from build123d import *

# Parameters (mm, degrees)
F1_DEPTH = 32.3
F2_W     = 34
F2_H     = 43.9928
F3_DEPTH = 4.2
F4_R     = 1.8
F5_DEPTH = 25.4


with BuildPart() as f1:
    # F0 (on Top) → F1 (new body)
    with BuildSketch(Plane.XY):
        with BuildLine():
            Line((-13.075, -13.5), (13.075, -13.5))
            ThreePointArc((13.075, -13.5), (14.842766953, -12.767766953), (15.575, -11))
            Line((15.575, -11), (15.575, 11))
            ThreePointArc((15.575, 11), (14.842766953, 12.767766953), (13.075, 13.5))
            Line((13.075, 13.5), (-13.075, 13.5))
            ThreePointArc((-13.075, 13.5), (-14.842766953, 12.767766953), (-15.575, 11))
            Line((-15.575, 11), (-15.575, -11))
            ThreePointArc((-15.575, -11), (-14.842766953, -12.767766953), (-13.075, -13.5))
        make_face()
    extrude(amount=F1_DEPTH)

    # F2 (on face) → F3 (join)
    with BuildSketch(Plane.XY.offset(32.3)):
        Rectangle(F2_W, F2_H)
        with BuildLine():
            Line((-15.575, -11), (-15.575, 11))
            ThreePointArc((-15.575, 11), (-14.842766953, 12.767766953), (-13.075, 13.5))
            Line((-13.075, 13.5), (13.075, 13.5))
            ThreePointArc((13.075, 13.5), (14.842766953, 12.767766953), (15.575, 11))
            Line((15.575, 11), (15.575, -11))
            ThreePointArc((15.575, -11), (14.842766953, -12.767766953), (13.075, -13.5))
            Line((13.075, -13.5), (-13.075, -13.5))
            ThreePointArc((-13.075, -13.5), (-14.842766953, -12.767766953), (-15.575, -11))
        make_face(mode=Mode.SUBTRACT)
        with BuildLine():
            ThreePointArc((-13.075, 13.5), (-14.842766953, 12.767766953), (-15.575, 11))
            Line((-15.575, 11), (-15.575, -11))
            ThreePointArc((-15.575, -11), (-14.842766953, -12.767766953), (-13.075, -13.5))
            Line((-13.075, -13.5), (13.075, -13.5))
            ThreePointArc((13.075, -13.5), (14.842766953, -12.767766953), (15.575, -11))
            Line((15.575, -11), (15.575, 11))
            ThreePointArc((15.575, 11), (14.842766953, 12.767766953), (13.075, 13.5))
            Line((13.075, 13.5), (-13.075, 13.5))
        make_face()
    extrude(amount=F3_DEPTH)

    # F4 (on face) → F5 (cut)
    with BuildSketch(Plane.XY.offset(36.5)):
        with Locations((0, 18.0036)):
            Circle(F4_R)
        with Locations((0, -17.9964)):
            Circle(F4_R)
    extrude(amount=-F5_DEPTH, mode=Mode.SUBTRACT)


solid = f1.part
Can you work these out from the model? Positions are in its coordinate system, mm. A direction names the side the tool comes from. Coordinates: 2 decimals unless noted, no trailing zeros. Loops run counter-clockwise (first coordinate to the right, second up) from the corner with the lowest first, then second, coordinate; pieces in that order, holes last. Notation, with made-up numbers: (75, 3.5) - (114, 3.5) arc R15 cw to (114, 28.5) - close; hole circle Ø6 at (15, 88.5). An arc over 180 degrees is marked (long way). Answer as a JSON object with one key per item and string values. Group by question number.
Item 1: If I drill on L1, parallel to Y at x = 0, z = 34.6; L2, parallel to Z at x = -1.5, y = 16; L3, parallel to Y at x = 1.5, z = 28.5, over which ranges is the centre line in solid material (lowest first)? Write a range as from..to.
Item 2: On a 3-axis mill with a long thin cutter (end or side, diameter ignored), from which of +Z, -Z, +X, -X, +Y, -Y can I reach the whole of each face in a straight line? I mean faces 4 (the face through (14.82, -12.79, 15.92)), 5 (the face through (0, -13.5, 16)), 6 (the face through (0, 13.5, 16)), 7 (the face through (-15.575, 0, 16)), 8 (the face through (15.575, 0, 16)). Say none if no direction works.
Item 3: If we section it at C-C (z = 11): List the corners of the cut face in (x, y) for me (3 decimals), plus the area to 3 significant figures.
Item 4: For pin 1 (1 mm diameter, centred on x = 11.5, z = 28.5, fed in from -Y); pin 2 (8 mm diameter, centred on y = 12.5, z = 19.5, fed in from -X) (3 decimals); pin 3 (1.5 mm diameter, centred on x = -0.5, z = 24.5, fed in from +Y), each with a flat end and sliding along its axis, tell me the tip position at first contact or that it passes through.
Item 5: If we section it at A-A (x = 0): List the corners of the cut face in (y, z) for me.
Item 6: If we mould it in two halves opening along X, with no side actions, what happens to faces 1 (the face through (17, 0, 34)), 2 (the face through (0, 15, 32.3)), 3 (the face through (-0.23, -16.21, 34.43))? For each: released by +X, released by -X, zero draft, split by the parting line, or undercut.
Item 7: If we section it at B-B (x = 12.5): List the corners of the cut face in (y, z) for me, plus the area to 3 significant figures.
Returned:
{
 "1": {"L1": "y = -22..-19.8, -16.2..16.2, 19.8..22", "L2": "z = 32.3..36.5", "L3": "y = -13.5..13.5"},
 "2": {"face 4": "-Z, +X, -Y", "face 5": "-Z, +X, -X, -Y", "face 6": "-Z, +X, -X, +Y", "face 7": "-Z, -X, +Y, -Y", "face 8": "-Z, +X, +Y, -Y"},
 "3": {"outline": "(-15.575, -11) arc R2.5 ccw to (-13.075, -13.5) - (13.075, -13.5) arc R2.5 ccw to (15.575, -11) - (15.575, 11) arc R2.5 ccw to (13.075, 13.5) - (-13.075, 13.5) arc R2.5 ccw to (-15.575, 11) - close", "area": "836 mm²"},
 "4": {"pin 1": "stops at y = -13.5", "pin 2": "stops at x = -15.575", "pin 3": "stops at y = 13.5"},
 "5": {"outline": "(-22, 32.3) - (-19.8, 32.3) - (-19.8, 36.5) - (-22, 36.5) - close; (-16.2, 32.3) - (-13.5, 32.3) - (-13.5, 0) - (13.5, 0) - (13.5, 32.3) - (16.2, 32.3) - (16.2, 36.5) - (-16.2, 36.5) - close; (19.8, 32.3) - (22, 32.3) - (22, 36.5) - (19.8, 36.5) - close"},
 "6": {"face 1": "released by +X", "face 2": "zero draft", "face 3": "undercut"},
 "7": {"outline": "(-22, 32.3) - (-13.5, 32.3) - (-13.5, 0) - (13.5, 0) - (13.5, 32.3) - (22, 32.3) - (22, 36.5) - (-22, 36.5) - close", "area": "1,060 mm²"}
}
